Design review of the part built by this model. Coordinates are the model's own, in mm. A direction names the side the tool comes from. Give positions to 0.01 mm unless a question says otherwise; leave off trailing zeros. Loops run counter-clockwise (first coordinate to the right, second up) from the corner with the lowest first, then second, coordinate; pieces in that order, holes last. Notation, with made-up numbers: M -31,-4.5 L 17,-4.5 A6 cw 17,6.5 Z; hole C 62,37.5 d3. An arc over 180 degrees is marked long. Use a Markdown table: item, result. Add a question column.
(1) Insertion check: pin 1 Ø6 at (x, z) = (-3, -14.5) entering from +Y; pin 2 Ø6 at (x, y) = (-14.5, -17) entering from +Z; pin 3 Ø4.5 at (x, y) = (12.77, 7.38) entering from +Z. Each pin has a flat end and moves straight along its axis. Give the tip position at first contact, or say it passes through.
(2) Draft analysis for pull direction X (two halves, no side actions). For faces 3 (the face through (11.21, -24.35, 13.47)), 4 (the face through (0, -30.5, 0)), 5 (the face through (-11.766, -24.354, -12.403)), 6 (the face through (19.1, -26.06, 19.14)), state which applies: pulls with the +X half, pulls with the -X half, needs draft (parallel to the pull), parting line crosses it, or undercut.
(3) Add section C-C, the plane z = -14.5. Give the boundary of the cut face in (x, y), then the cut area to 3 significant figures.
(4) For probe 1 along Y at (x, z) = (15.5, 3); probe 2 along X at (y, z) = (-15.5, 0); probe 3 along Y at (x, z) = (-0.5, 6.5), list the stretches that pass through material, from the lowest coordinate up.
(5) Add section B-B, the plane x = 0. Give the boundary of the cut face in (y, z).
(6) For faces 1 (the face through (-2.38, -10.74, 0.11)), 2 (the face through (0, -21.5, 14)), list the 3-axis set-ups (+Z, -Z, +X, -X, +Y, -Y) from which the entire face can be reached by the end or side of a thin tool; tool diameter is ignored.
(7) Add section D-D, the plane y = 0. Give the boundary of the cut face in (x, z), then the cut area to 3 significant figures.
(8) Add section A-A, the plane y = -15.5. Give the boundary of the cut face in (x, z).
```python
from build123d import *

# Parameters (mm, degrees)
SKETCH_1_W                 = 40
SKETCH_1_H                 = 43
EXTRUDE_284_DEPTH          = 7.5
NEMA17_M3_D                = 3.4
NEMA17_M3_CSINK_D          = 6.3
NEMA17_M3_CSINK_ANGLE      = 90
SKETCH_8_R                 = 11
CUT_EXTRUDE_1_DEPTH        = 33.973474188
SKETCH_12_W                = 40
SKETCH_12_H                = 40
EXTRUDE_1_DEPTH            = 9
FILLET_1_R                 = 3
HOLE_WIZARD_M6_D           = 6.6
HOLE_WIZARD_M6_CSINK_D     = 12.6
HOLE_WIZARD_M6_CSINK_ANGLE = 90
HOLE_WIZARD_M3_D           = 3.4
HOLE_WIZARD_M3_CSINK_D     = 6.3
HOLE_WIZARD_M3_CSINK_ANGLE = 90


with BuildPart() as part:
    # Эскиз1 → Extrude 284 (new, symmetric)
    with BuildSketch(Plane.XY):
        Rectangle(SKETCH_1_W, SKETCH_1_H)
    extrude(amount=EXTRUDE_284_DEPTH, both=True)

    # КреплениеNema17-M3 (through all)
    with Locations(Plane(origin=(0, 0, -7.5), x_dir=(-1, 0, 0), z_dir=(0, 0, -1))):
        with Locations((-15.5, 15.5), (15.5, 15.5), (15.5, -15.5), (-15.5, -15.5)):
            CounterSinkHole(NEMA17_M3_D / 2, NEMA17_M3_CSINK_D / 2, counter_sink_angle=NEMA17_M3_CSINK_ANGLE)

    # Эскиз8 → Вырез1 (cut, through all)
    with BuildSketch(Plane.XY.offset(7.5)):
        Circle(SKETCH_8_R)
    extrude(amount=-CUT_EXTRUDE_1_DEPTH, mode=Mode.SUBTRACT)

    # Эскиз12 → Бобышка-Вытянуть1 (add)
    with BuildSketch(Plane.XZ.offset(21.5)):
        Rectangle(SKETCH_12_W, SKETCH_12_H)
    extrude(amount=EXTRUDE_1_DEPTH)

    # Скругление1
    fillet_1_edges = [part.edges().sort_by_distance(p)[0] for p in [
        (-20, -26, 20),
        (-20, -26, -20),
        (20, -26, -20),
        (20, -26, 20),
    ]]
    fillet(fillet_1_edges, radius=FILLET_1_R)

    # КреплениеКронштейна-M6 (through all)
    with Locations(Plane(origin=(0, -21.5, 0), x_dir=(1, 0, 0), z_dir=(0, 1, 0))):
        with Locations((-14.5, -14.5), (14.5, -14.5), (14.5, 14.5), (-14.5, 14.5)):
            CounterSinkHole(HOLE_WIZARD_M6_D / 2, HOLE_WIZARD_M6_CSINK_D / 2, counter_sink_angle=HOLE_WIZARD_M6_CSINK_ANGLE)

    # КреплениеБлокаПодшипниковM3 (through all)
    with Locations(Plane.XY.offset(7.5)):
        with Locations((-12.773874706, 7.375), (12.773874706, 7.375), (12.773874706, -7.375), (-12.773874706, -7.375)):
            CounterSinkHole(HOLE_WIZARD_M3_D / 2, HOLE_WIZARD_M3_CSINK_D / 2, counter_sink_angle=HOLE_WIZARD_M3_CSINK_ANGLE)


solid = part.part
```
Established:
| question | item | result |
|---|---|---|
| 1 | pin 1 | y = -21.5 |
| 1 | pin 2 | z = 7.5 |
| 1 | pin 3 | z = 6.61 |
| 2 | face 3 | undercut |
| 2 | face 4 | needs draft |
| 2 | face 5 | undercut |
| 2 | face 6 | pulls with the +X half |
| 3 | outline | M -20,-30.5 L -17.8,-30.5 L -17.8,-24.5 L -20,-22.3 Z; M -11.2,-30.5 L 11.2,-30.5 L 11.2,-24.5 L 8.2,-21.5 L -8.2,-21.5 L -11.2,-24.5 Z; M 17.8,-30.5 L 20,-30.5 L 20,-22.3 L 17.8,-24.5 Z |
| 3 | area | 224 mm^2 |
| 4 | probe 1 | -30.5 to -17.2, -13.8 to 13.8, 17.2 to 21.5 |
| 4 | probe 2 | -20 to -17.2, -13.8 to 13.8, 17.2 to 20 |
| 4 | probe 3 | -30.5 to -10.99, 10.99 to 21.5 |
| 5 | outline | M -30.5,-20 L -21.5,-20 L -21.5,-7.5 L -11,-7.5 L -11,7.5 L -21.5,7.5 L -21.5,20 L -30.5,20 Z; M 11,-7.5 L 21.5,-7.5 L 21.5,7.5 L 11,7.5 Z |
| 6 | face 1 | +Z, -Z |
| 6 | face 2 | +Z, +X, -X, +Y |
| 7 | outline | M -20,-7.5 L -11,-7.5 L -11,7.5 L -20,7.5 Z; M 11,-7.5 L 20,-7.5 L 20,7.5 L 11,7.5 Z |
| 7 | area | 270 mm^2 |
| 8 | outline | M -20,-7.5 L -18.65,-7.5 L -17.2,-6.05 L -17.2,7.5 L -20,7.5 Z; M -13.8,-6.05 L -12.35,-7.5 L 12.35,-7.5 L 13.8,-6.05 L 13.8,7.5 L -13.8,7.5 Z; M 17.2,-6.05 L 18.65,-7.5 L 20,-7.5 L 20,7.5 L 17.2,7.5 Z |
